```python
from build123d import *

# Parameters (mm, degrees)
SKETCH_1_W      = 10
SKETCH_1_H      = 10
SKETCH_1_W_2    = 25
EXTRUDE_1_DEPTH = 200


with BuildPart() as part:
    # Эскиз1 → Бобышка-Вытянуть1 (new body)
    with BuildSketch(Plane(origin=(0, 0, 0), x_dir=(1, 0, 0), z_dir=(0, 1, 0))):
        Polygon((-5, 40), (-5, 2), (0, 40), align=None)
        Polygon((0, 40), (-5, 2), (-5, -30), (5, -30), (5, 40), align=None)
        with Locations((0, -35)):
            Rectangle(SKETCH_1_W, SKETCH_1_H)
        Polygon((-5, -40), (-5, -30), (-20, -30), (-20, -60), (5, -60), (5, -40), align=None)
        with Locations((17.5, -35)):
            Rectangle(SKETCH_1_W_2, SKETCH_1_H)
    extrude_1 = extrude(amount=EXTRUDE_1_DEPTH)

    # Зеркальное отражение1: Бобышка-Вытянуть1 across plane
    add(extrude_1.mirror(Plane(origin=(-20, 200, 30), x_dir=(0, 0, 1), z_dir=(1, 0, 0))))


solid = part.part
```
Can you work these out from the model? Positions are in its coordinate system, mm. A direction names the side the tool comes from. Coordinates: 2 decimals unless noted, no trailing zeros. Loops run counter-clockwise (first coordinate to the right, second up) from the corner with the lowest first, then second, coordinate; pieces in that order, holes last. Notation, with made-up numbers: (-21, -6.75) -> (13, -6.75) arc R19 cw to (13, 11.25) -> close; hole circle Ø2 at (-19, 29.5). An arc over 180 degrees is marked (long way). Put each result on its own line as item: value. Start each with the question number.
Q1. I'm going to push flat-ended pins straight in: P1, Ø1.5, axis at y = 96, z = -12, coming from the +X side; P2, Ø16, axis at y = 73, z = 53.5, coming from the -X side; P3, Ø20, axis at x = -59, y = 92.5, coming from the +Z side. Where does each tip first touch, or does it pass through?
Q2. For faces 1 (the face through (-20, 99, 30)), 2 (the face through (-57, 99, 30)), 3 (the face through (17, 99, 30)), which set-ups out of +Z, -Z, +X, -X, +Y, -Y let a thin tool reach every point of the face, with its end or its side?
Q3. I want a section at B-B (y = 24). Write out the boundary of the cut face in (x, z), plus the area to 3 significant figures.
Q4. I want a section at A-A (z = 7). Write out the boundary of the cut face in (x, y).
Q5. Thinking about a two-plate mould opening in X: for faces 4 (the face through (5, 99, -5)), 5 (the face through (-5, 99, -5)), 6 (the face through (-45, 99, -5)), which applies, pulls with the +X half, pulls with the -X half, needs draft (parallel to the pull), parting line crosses it, or undercut?
Q6. If I drill on line 1 (X direction, y = 74, z = 6.5); line 2 (Z direction, x = -33, y = 14.5); line 3 (X direction, y = 98, z = 41), over which ranges is the centre line in solid material (lowest first)? Write a range as [from, to].
Q7. I want a section at D-D (z = 44). Write out the boundary of the cut face in (x, y), plus the area to 3 significant figures.
Q8. I want a section at C-C (x = -22.5). Write out the boundary of the cut face in (y, z).
Taken from the geometry:
1. P1: stops at x = 5
1. P2: stops at x = -45
1. P3: stops at z = 40
2. face 1: -Z, +Y, -Y
2. face 2: -Z, -X, +Y, -Y
2. face 3: -Z, +X, +Y, -Y
3. outline: (-70, 30) -> (-45, 30) -> (-45, -40) -> (-35, -40) -> (-35, 30) -> (-5, 30) -> (-5, -40) -> (5, -40) -> (5, 30) -> (30, 30) -> (30, 40) -> (5, 40) -> (5, 60) -> (-45, 60) -> (-45, 40) -> (-70, 40) -> close
3. area: 3,400 mm2
4. outline: (-45, 0) -> (-35, 0) -> (-35, 200) -> (-45, 200) -> close; (-5, 0) -> (5, 0) -> (5, 200) -> (-5, 200) -> close
5. face 4: pulls with the +X half
5. face 5: undercut
5. face 6: pulls with the -X half
6. line 1: x = [-45, -35], [-5, 5]
6. line 2: z = [30, 60]
6. line 3: x = [-45, 5]
7. outline: (-45, 0) -> (5, 0) -> (5, 200) -> (-45, 200) -> close
7. area: 10,000 mm2
8. outline: (0, 30) -> (200, 30) -> (200, 60) -> (0, 60) -> close
